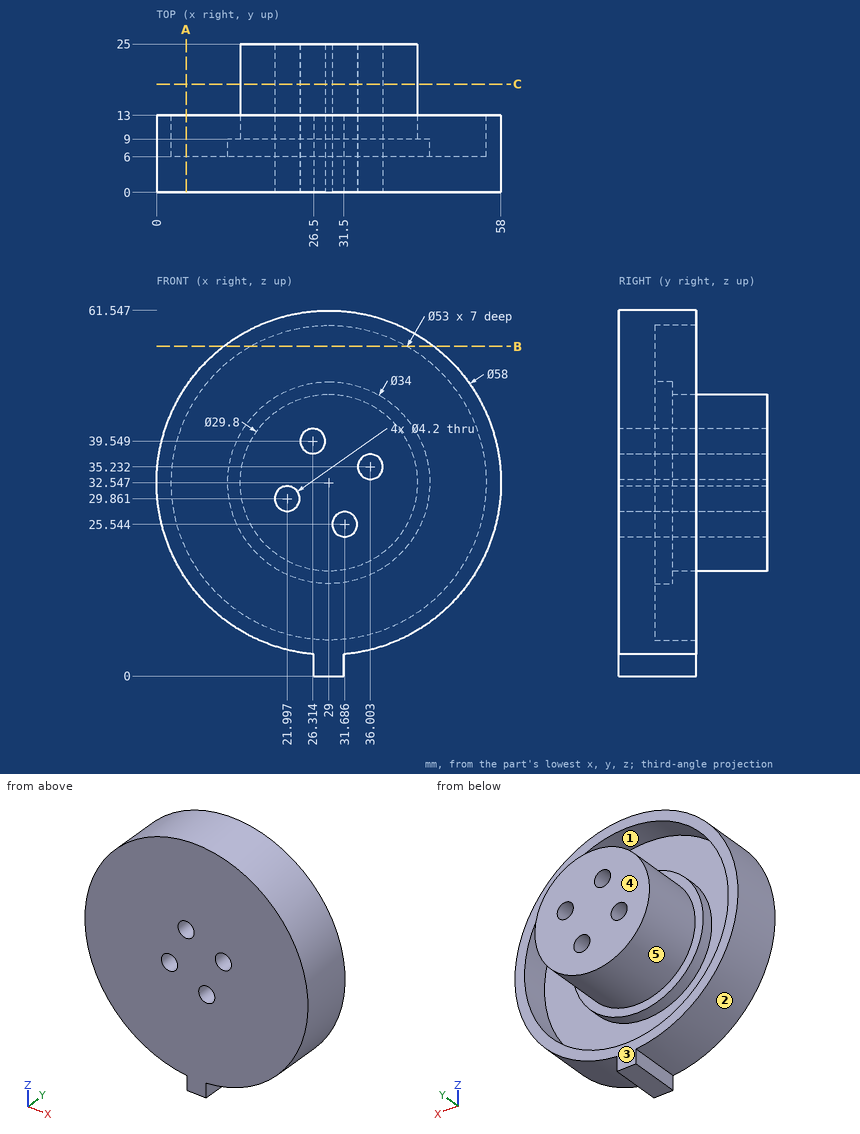
Input: dimensioned drawing with shaded views. Units: mm. Origin: part minimum x, y, z. A direction names the side the tool comes from. Coordinates: 2 decimals unless noted, no trailing zeros. Order: outer loops, then holes, each group sorted by start corner. A loop starts at its lowest first (then second) coordinate and runs counter-clockwise, first axis right, second up.
1. Contact query for flat-ended pins moving along their axis: P1, Ø8, axis at y = 18, z = 15.5, coming from the -X side (1 decimal); P2, Ø6, axis at x = 51, z = 19, coming from the +Y side; P3, Ø4, axis at x = 21.5, y = 18, coming from the +Z side (1 decimal). Output: stop coordinate, or through.
Checked values:
P1: stops at x = 21.8
P2: stops at y = 13
P3: stops at z = 46.4
2. Draft query along X for the marked faces 1, 2 and 3. Return one class per face: +X half, -X half, draft (parallel to the pull), parting line (faces both ways), or undercut.
Checked values:
face 1: undercut
face 2: parting line
face 3: draft
3. Cut plane A-A, the plane x = 5. Return loops of the section in (y, z) (1 decimal), plus the area to 3 significant figures.
Checked values:
outline: (0, 16.3) - (13, 16.3) - (13, 21.3) - (6, 21.3) - (6, 43.8) - (13, 43.8) - (13, 48.8) - (0, 48.8) - close
area: 266 mm2
4. Cut plane B-B, the plane z = 55.5. Return loops of the section in (x, y).
Checked values:
outline: (11.28, 0) - (46.72, 0) - (46.72, 13) - (42.24, 13) - (42.24, 6) - (15.76, 6) - (15.76, 13) - (11.28, 13) - close
5. Cut plane C-C, the plane y = 18.25. Count the separate pieces of the cut face and the enclosed holes in it, plus the area to 3 significant figures.
Checked values:
separate pieces: 1
enclosed holes: 4
area: 642 mm2
6. Ray query, line 1 along Z through (x, y) = (22, 9.5) (1 decimal); line 2 along Y through (x, z) = (40.5, 56); line 3 along Y through (x, z) = (30, 3.5). Return the intervals inside material, ascending.
Checked values:
line 1: z = 4.4 to 7, 19.4 to 27.8, 32 to 45.7, 58.1 to 60.7
line 2: y = 0 to 6
line 3: y = 0 to 13
7. Access query for the marked faces 4 and 5. Directions: +Z, -Z, +X, -X, +Y, -Y. A direction counts if a zero-diameter tool reaches every point of the face in a straight line with its end or side. Return the directions, or none.
Checked values:
face 4: +Z, -Z, +X, -X, +Y
face 5: +Y
